Check sheet for the modelled part. Datum: model origin and axes. Units: mm. A direction names the side the tool comes from. Round coordinates to 2 decimals unless told otherwise and drop trailing zeros. Return JSON: item names as keys, results as strings.
from build123d import *

# Parameters (mm, degrees)
BOSS_EXTRUDE1_DEPTH = 3
SKETCH2_W           = 107
SKETCH2_H           = 20
CUT_EXTRUDE1_DEPTH  = 143.254173928
SKETCH3_R           = 26
CUT_EXTRUDE2_DEPTH  = 143.254173928
FILLET1_R           = 5
SKETCH4_W           = 30.4
SKETCH4_H           = 116.319851171
CUT_EXTRUDE3_DEPTH  = 143.254173928
SKETCH5_W           = 52
SKETCH5_H           = 70
CUT_EXTRUDE4_DEPTH  = 143.254173928
FILLET2_R           = 10
FILLET3_R           = 2
SKETCH6_W           = 28
SKETCH6_H           = 50
BOSS_EXTRUDE2_DEPTH = 3
FILLET4_R           = 3
SKETCH7_R           = 2.1
CUT_EXTRUDE5_DEPTH  = 143.254174065
SKETCH8_R           = 2.6
CUT_EXTRUDE6_DEPTH  = 143.254174065


with BuildPart() as part:
    # Sketch1 → Boss-Extrude1 (new body)
    with BuildSketch(Plane.XY):
        Polygon((-65, 106.5), (-65, -126.5), (65, -126.5), (65, 126.5), (-42, 126.5), (-42, 106.5), align=None)
    extrude(amount=BOSS_EXTRUDE1_DEPTH)

    # Sketch2 → Cut-Extrude1 (cut, through all)
    with BuildSketch(Plane.XY.offset(3)):
        with Locations((11.5, 116.5)):
            Rectangle(SKETCH2_W, SKETCH2_H)
    extrude(amount=-CUT_EXTRUDE1_DEPTH, mode=Mode.SUBTRACT)

    # Sketch3 → Cut-Extrude2 (cut, through all)
    with BuildSketch(Plane(origin=(0, 0, 0), x_dir=(-1, 0, 0), z_dir=(0, 0, -1))):
        with Locations((0, -6.5)):
            Circle(SKETCH3_R)
    extrude(amount=-CUT_EXTRUDE2_DEPTH, mode=Mode.SUBTRACT)

    # Fillet1
    fillet1_edges = [part.edges().sort_by_distance(p)[0] for p in [
        (65, -126.5, 1.5),
        (-65, -126.5, 1.5),
        (-65, 106.5, 1.5),
        (65, 106.5, 1.5),
    ]]
    fillet(fillet1_edges, radius=FILLET1_R)

    # Sketch4 → Cut-Extrude3 (cut, through all)
    with BuildSketch(Plane.XY.offset(3)):
        with Locations((0, -63.840074415)):
            Rectangle(SKETCH4_W, SKETCH4_H)
    extrude(amount=-CUT_EXTRUDE3_DEPTH, mode=Mode.SUBTRACT)

    # Sketch5 → Cut-Extrude4 (cut, through all)
    with BuildSketch(Plane(origin=(0, 0, 0), x_dir=(-1, 0, 0), z_dir=(0, 0, -1))):
        with Locations((0, 28.5)):
            Rectangle(SKETCH5_W, SKETCH5_H)
    extrude(amount=-CUT_EXTRUDE4_DEPTH, mode=Mode.SUBTRACT)

    # Fillet2
    fillet2_edges = [part.edges().sort_by_distance(p)[0] for p in [
        (26, 63.5, 1.5),
        (-26, 63.5, 1.5),
    ]]
    fillet(fillet2_edges, radius=FILLET2_R)

    # Fillet3
    fillet3_edges = [part.edges().sort_by_distance(p)[0] for p in [
        (-15.2, -27.594074997, 1.5),
        (15.2, -27.594074997, 1.5),
        (-15.2, -122, 1.5),
        (15.2, -122, 1.5),
    ]]
    fillet(fillet3_edges, radius=FILLET3_R)

    # Sketch6 → Boss-Extrude2 (add)
    with BuildSketch(Plane(origin=(0, 0, 0), x_dir=(-1, 0, 0), z_dir=(0, 0, -1))):
        with Locations((0, 63.5)):
            Rectangle(SKETCH6_W, SKETCH6_H)
    extrude(amount=-BOSS_EXTRUDE2_DEPTH)

    # Fillet4
    fillet4_edges = [part.edges().sort_by_distance(p)[0] for p in [
        (14, 38.5, 1.5),
        (-14, 38.5, 1.5),
        (-14, 63.5, 1.5),
        (14, 63.5, 1.5),
    ]]
    fillet(fillet4_edges, radius=FILLET4_R)

    # Sketch7 → Cut-Extrude5 (cut, through all)
    with BuildSketch(Plane(origin=(0, 0, 0), x_dir=(-1, 0, 0), z_dir=(0, 0, -1))):
        with Locations((-55, 90)):
            Circle(SKETCH7_R)
        with Locations((-55, 50)):
            Circle(SKETCH7_R)
        with Locations((-55, 10)):
            Circle(SKETCH7_R)
        with Locations((-55, -30)):
            Circle(SKETCH7_R)
        with Locations((-55, -70)):
            Circle(SKETCH7_R)
        with Locations((-55, -110)):
            Circle(SKETCH7_R)
    cut_extrude5 = extrude(amount=-CUT_EXTRUDE5_DEPTH, mode=Mode.SUBTRACT)

    # Mirror1: Cut-Extrude5 across plane
    add(cut_extrude5.mirror(Plane(origin=(0, 0, 0), x_dir=(0, 0, 1), z_dir=(1, 0, 0))), mode=Mode.SUBTRACT)

    # Sketch8 → Cut-Extrude6 (cut, through all)
    with BuildSketch(Plane.XY.offset(3)):
        with Locations((-1.1e-08, 49.569851171)):
            Circle(SKETCH8_R)
        with Locations((-1.1e-08, 85.569851171)):
            Circle(SKETCH8_R)
    extrude(amount=-CUT_EXTRUDE6_DEPTH, mode=Mode.SUBTRACT)


solid = part.part
Q1. Material ranges on line 1 (Y direction, x = 0, z = 2.35); line 2 (X direction, y = -33.5, z = 2.2); line 3 (X direction, y = 18.5, z = 1.4), recorded low to high.
Results list:
{"line 1": "-126.5 to -122, 38.5 to 46.97, 52.17 to 82.97, 88.17 to 106.5", "line 2": "-65 to -15.2, 15.2 to 65", "line 3": "-65 to -26, 26 to 65"}
Q2. Section check A-A (z = 1.5). Count the separate pieces of the cut face and the enclosed holes in it, then the cut area to 3 significant figures.
Results list:
{"separate pieces": "1", "enclosed holes": "15", "area": "23,300 mm^2"}
Q3. Tool access check on faces 4 (the cylindrical face through (-23.493, 60.122, 1.521)), 5 (the cylindrical face through (-63.57, 105, 1.52)). Record the directions out of +Z, -Z, +X, -X, +Y, -Y that give a thin tool (end or side, any length) a straight path to the whole face; none if there is none.
Results list:
{"face 4": "+Z, -Z", "face 5": "+Z, -Z, -X, +Y"}
Q4. Draft check along Y on faces 1 (the cylindrical face through (63.5, 105.07, 1.48)), 2 (the cylindrical face through (-63.57, -125, 1.52)), 3 (the cylindrical face through (53.06, -30.8, 1.48)). Enter one of: released by +Y, released by -Y, zero draft, split by the parting line, or undercut.
Results list:
{"face 1": "released by +Y", "face 2": "released by -Y", "face 3": "undercut"}
